from build123d import *

# Parameters (mm, degrees)
SKETCH1_R           = 44
BOSS_EXTRUDE1_DEPTH = 2
SKETCH2_W           = 44
SKETCH2_H           = 88
BOSS_EXTRUDE2_DEPTH = 2
SKETCH3_R           = 1.75
CUT_EXTRUDE1_DEPTH  = 3
CIRPATTERN1_COUNT   = 8
SKETCH4_R           = 37.5
CUT_EXTRUDE2_DEPTH  = 3
FILLET1_R           = 10


with BuildPart() as part:
    # Sketch1 → Boss-Extrude1 (new body)
    with BuildSketch(Plane(origin=(0, 0, 0), x_dir=(1, 0, 0), z_dir=(0, 1, 0))):
        Circle(SKETCH1_R)
    extrude(amount=BOSS_EXTRUDE1_DEPTH)

    # Sketch2 → Boss-Extrude2 (add)
    with BuildSketch(Plane(origin=(0, 2, 0), x_dir=(1, 0, 0), z_dir=(0, 1, 0))):
        with Locations((-22, 0)):
            Rectangle(SKETCH2_W, SKETCH2_H)
    extrude(amount=-BOSS_EXTRUDE2_DEPTH)

    # Sketch3 → Cut-Extrude1 (cut, through all)
    with BuildSketch(Plane(origin=(0, 2, 0), x_dir=(1, 0, 0), z_dir=(0, 1, 0))):
        with Locations((41, 0)):
            Circle(SKETCH3_R)
    cut_extrude1 = extrude(amount=-CUT_EXTRUDE1_DEPTH, mode=Mode.SUBTRACT)

    # CirPattern1: Cut-Extrude1 ×8 about axis
    cirpattern1_axis = Axis((0, 0, 0), (0, 1, 0))
    for i in range(1, CIRPATTERN1_COUNT):
        add(cut_extrude1.rotate(cirpattern1_axis, i * 360 / CIRPATTERN1_COUNT), mode=Mode.SUBTRACT)

    # Sketch4 → Cut-Extrude2 (cut, through all)
    with BuildSketch(Plane(origin=(0, 2, 0), x_dir=(1, 0, 0), z_dir=(0, 1, 0))):
        Circle(SKETCH4_R)
    extrude(amount=-CUT_EXTRUDE2_DEPTH, mode=Mode.SUBTRACT)

    # Fillet1
    fillet1_edges = [part.edges().sort_by_distance(p)[0] for p in [
        (-44, 1, 44),
        (-44, 1, -44),
    ]]
    fillet(fillet1_edges, radius=FILLET1_R)


solid = part.part
Can you work these out from the model? Positions are in its coordinate system, mm. Round coordinates to 2 decimals unless told otherwise and drop trailing zeros. Loops run counter-clockwise (first coordinate to the right, second up) from the corner with the lowest first, then second, coordinate; pieces in that order, holes last. Notation, with made-up numbers: (-27, 78) - (13, 78) arc R8 ccw to (13, 86) - close; hole circle Ø5 at (76, 62). An arc over 180 degrees is marked (long way). Write item = value, one per line. Start each with the question number.
(1) If I drill on probe 1 along X at (y, z) = (1.8, -23); probe 2 along Z at (x, y) = (-15.5, 0.9); probe 3 along X at (y, z) = (0.7, -33), over which ranges is the centre line in solid material (lowest first)? Write a range as [from, to].
(2) If we section it at B-B (x = 41): Please give me the cut outline in (y, z), and give its area (3 significant figures).
(3) If we section it at A-A (z = 0): Please give me the cut outline in (x, y), and give its area (3 significant figures).
(4) For P1, Ø5.5, axis at x = 0, z = 41, coming from the +Y side; P2, Ø8, axis at x = -21, z = -21, coming from the -Y side, each with a flat end and sliding along its axis, tell me the tip position at first contact or that it passes through.
(5) If we section it at D-D (y = 0.85): Give the number of separate pieces and of enclosed holes in the cut face, and give its area (3 significant figures).
(6) If we mould it in two halves opening along Z, with no side actions, what happens to faces 1 (the face through (-17, 1, 44)), 2 (the face through (-0.67, 1.014, 42.617)), 3 (the face through (-36, 0, -13))? For each: released by +Z, released by -Z, zero draft, split by the parting line, or undercut.
(7) If we section it at C-C (z = 41): Please give me the cut outline in (x, y), and give its area (3 significant figures).
Ans:
q1.probe_1 = [-44, -29.62], [29.62, 37.51]
q1.probe_2 = [-44, -34.15], [34.15, 44]
q1.probe_3 = [-44, -17.81], [17.81, 29.1]
q2.outline = (0, -15.97) - (2, -15.97) - (2, -1.75) - (0, -1.75) - close; (0, 1.75) - (2, 1.75) - (2, 15.97) - (0, 15.97) - close
q2.area = 56.9 mm²
q3.outline = (-44, 0) - (-42.75, 0) - (-42.75, 2) - (-44, 2) - close; (-39.25, 0) - (-37.5, 0) - (-37.5, 2) - (-39.25, 2) - close; (37.5, 0) - (39.25, 0) - (39.25, 2) - (37.5, 2) - close; (42.75, 0) - (44, 0) - (44, 2) - (42.75, 2) - close
q3.area = 12.0 mm²
q4.P1 = 2
q4.P2 = through
q5.separate_pieces = 1
q5.enclosed_holes = 9
q5.area = 2,380 mm²
q6.face_1 = released by +Z
q6.face_2 = undercut
q6.face_3 = zero draft
q7.outline = (-41.14, 0) - (-1.75, 0) - (-1.75, 2) - (-41.14, 2) - close; (1.75, 0) - (15.97, 0) - (15.97, 2) - (1.75, 2) - close
q7.area = 107 mm²
